```python
from build123d import *

# Parameters (mm, degrees)
F0_R     = 4.5
F0_R_2   = 3
F0_R_3   = 35
F1_DEPTH = 6.35


with BuildPart() as f1:
    # F0 (on Front) → F1 (new body, symmetric)
    with BuildSketch(Plane.XZ):
        with BuildLine():
            Line((32.5, 49), (-32.5, 49))
            ThreePointArc((-32.5, 49), (-37.198943, 47.675932), (-40.515282, 44.093318))
            Line((-40.515282, 44.093318), (-49.5, 26.5))
            Line((-49.5, 26.5), (-49.5, -30))
            Line((-49.5, -30), (-35.047059, -56))
            Line((-35.047059, -56), (35.047061, -56))
            Line((35.047061, -56), (41.142898, -35.010043))
            ThreePointArc((41.142898, -35.010043), (41.056204, -29.708696), (38, -25.376097))
            Line((38, -25.376097), (38, 25.376097))
            ThreePointArc((38, 25.376097), (40.577747, 28.531373), (41.5, 32.5))
            Line((41.5, 32.5), (41.5, 40))
            ThreePointArc((41.5, 40), (38.863961, 46.363961), (32.5, 49))
        make_face()
        with Locations((-32.5, -40)):
            Circle(F0_R, mode=Mode.SUBTRACT)
        with Locations((32.5, -32.5)):
            Circle(F0_R, mode=Mode.SUBTRACT)
        with Locations((-37.5, 22)):
            Circle(F0_R_2, mode=Mode.SUBTRACT)
        with Locations((-32.5, 40)):
            Circle(F0_R, mode=Mode.SUBTRACT)
        Circle(F0_R_3, mode=Mode.SUBTRACT)
        with Locations((32.5, 32.5)):
            Circle(F0_R, mode=Mode.SUBTRACT)
    extrude(amount=F1_DEPTH, both=True)


solid = f1.part
```
Can you work these out from the model? Positions are in its coordinate system, mm. A direction names the side the tool comes from. Give positions to 0.01 mm unless a question says otherwise; leave off trailing zeros. Loops run counter-clockwise (first coordinate to the right, second up) from the corner with the lowest first, then second, coordinate; pieces in that order, holes last. Notation, with made-up numbers: M 71,28 L 76,28 A16 cw 76,45 Z; hole C 81,79.5 d5. An arc over 180 degrees is marked long. Use CSV: the item, a comma, the result in double quotes. Start each with the question number.
1. Imagine slicing it at B-B, the plane y = -3. Write out the boundary of the cut face in (x, z), plus the area to 3 significant figures.
2. For P1, Ø8, axis at x = -32.5, z = 40, coming from the -Y side, with a flat end and sliding along its axis, tell me the tip position at first contact or that it passes through.
3. If we mould it in two halves opening along Z, with no side actions, what happens to faces 3 (the face through (40.552, -0.089, 28.48)), 4 (the face through (38.052, -0.089, -45.652)), 5 (the face through (41.5, 0, 36))? For each: released by +Z, released by -Z, zero draft, split by the parting line, or undercut.
4. On a 3-axis mill with a long thin cutter (end or side, diameter ignored), from which of +Z, -Z, +X, -X, +Y, -Y can I reach the whole of each face in a straight line? I mean faces 1 (the face through (38, 0, 0)), 2 (the face through (-30.42, 0.09, -43.99)). Say none if no direction works.
5. Imagine slicing it at C-C, the plane z = 22. Write out the boundary of the cut face in (x, y).
6. Imagine slicing it at D-D, the plane z = -17.5. Write out the boundary of the cut face in (x, y), plus the area to 3 significant figures.
7. Imagine slicing it at A-A, the plane x = 0. Write out the boundary of the cut face in (y, z).
8. If I drill on L1, parallel to Z at x = 29, y = 4.25; L2, parallel to Z at x = -30, y = 2; L3, parallel to Z at x = 4.5, y = -2.25, over which ranges is the centre line in solid material (lowest first)?
Response values:
1,outline,"M -49.5,-30 L -35.05,-56 L 35.05,-56 L 41.14,-35.01 A9 ccw 38,-25.38 L 38,25.38 A9 ccw 41.5,32.5 L 41.5,40 A9 ccw 32.5,49 L -32.5,49 A9 ccw -40.52,44.09 L -49.5,26.5 Z; hole C -37.5,22 d6; hole C -32.5,-40 d9; hole C -32.5,40 d9; hole C 0,0 d70; hole C 32.5,-32.5 d9; hole C 32.5,32.5 d9"
1,area,"4,820 mm^2"
2,P1,"through"
3,face 3,"undercut"
3,face 4,"released by -Z"
3,face 5,"zero draft"
4,face 1,"+X, +Y, -Y"
4,face 2,"+Y, -Y"
5,outline,"M -49.5,-6.35 L -40.5,-6.35 L -40.5,6.35 L -49.5,6.35 Z; M -34.5,-6.35 L -27.22,-6.35 L -27.22,6.35 L -34.5,6.35 Z; M 27.22,-6.35 L 38,-6.35 L 38,6.35 L 27.22,6.35 Z"
6,outline,"M -49.5,-6.35 L -30.31,-6.35 L -30.31,6.35 L -49.5,6.35 Z; M 30.31,-6.35 L 38,-6.35 L 38,6.35 L 30.31,6.35 Z"
6,area,"341 mm^2"
7,outline,"M -6.35,-56 L 6.35,-56 L 6.35,-35 L -6.35,-35 Z; M -6.35,35 L 6.35,35 L 6.35,49 L -6.35,49 Z"
8,L1,"-56 to -35.33, -29.67 to -19.6, 19.6 to 29.67, 35.33 to 49"
8,L2,"-56 to -43.74, -36.26 to -18.03, 18.03 to 36.26, 43.74 to 49"
8,L3,"-56 to -34.71, 34.71 to 49"
